Build history of the part. All positions in model axes, mm. A direction names the side the tool comes from. Round coordinates to 2 decimals unless told otherwise and drop trailing zeros. Loops run counter-clockwise (first coordinate to the right, second up) from the corner with the lowest first, then second, coordinate; pieces in that order, holes last.
from build123d import *

# Parameters (mm, degrees)
SALIENTE_EXTRUIR1_DEPTH = 304.8
CROQUIS4_R              = 15.875
SALIENTE_EXTRUIR2_DEPTH = 50.8
CROQUIS5_R              = 15.875
SALIENTE_EXTRUIR3_DEPTH = 25.4


with BuildPart() as part:
    # Croquis2 → Saliente-Extruir1 (new body)
    with BuildSketch(Plane.XY):
        Polygon((-63.5, 0), (-31.75, -54.99261314), (31.75, -54.99261314), (63.5, 0), (31.75, 54.99261314), (-31.75, 54.99261314), align=None)
    extrude(amount=-SALIENTE_EXTRUIR1_DEPTH)

    # Croquis4 → Saliente-Extruir2 (add)
    with BuildSketch(Plane.XY):
        Circle(CROQUIS4_R)
    extrude(amount=SALIENTE_EXTRUIR2_DEPTH)

    # Croquis5 → Saliente-Extruir3 (add)
    with BuildSketch(Plane(origin=(0, 0, -304.8), x_dir=(-1, 0, 0), z_dir=(0, 0, -1))):
        Circle(CROQUIS5_R)
    extrude(amount=SALIENTE_EXTRUIR3_DEPTH)


solid = part.part
(1) Slice it at B-B on z = -233. List the corners of the cut face in (x, y).
Responses:
outline: (-63.5, 0) - (-31.75, -54.99) - (31.75, -54.99) - (63.5, 0) - (31.75, 54.99) - (-31.75, 54.99) - close
(2) Slice it at A-A on x = 0. List the corners of the cut face in (y, z) (3 decimals), plus the area to 3 significant figures.
Responses:
outline: (-54.993, -304.8) - (-15.875, -304.8) - (-15.875, -330.2) - (15.875, -330.2) - (15.875, -304.8) - (54.993, -304.8) - (54.993, 0) - (15.875, 0) - (15.875, 50.8) - (-15.875, 50.8) - (-15.875, 0) - (-54.993, 0) - close
area: 35,900 mm2
(3) Slice it at C-C on y = 5.5. List the corners of the cut face in (x, z), plus the area to 3 significant figures.
Responses:
outline: (-60.32, -304.8) - (-14.89, -304.8) - (-14.89, -330.2) - (14.89, -330.2) - (14.89, -304.8) - (60.32, -304.8) - (60.32, 0) - (14.89, 0) - (14.89, 50.8) - (-14.89, 50.8) - (-14.89, 0) - (-60.32, 0) - close
area: 39,000 mm2
(4) Pin check, flat tips, straight feed: P1, Ø1.5, axis at y = 32, z = -75.5, coming from the +X side; P2, Ø1.5, axis at x = 36.5, z = -157.5, coming from the +Y side; P3, Ø5, axis at x = -35.5, y = -9, coming from the +Z side. Stop position of each tip, or through.
Responses:
P1: stops at x = 45.46
P2: stops at y = 48.06
P3: stops at z = 0
(5) Slice it at D-D on y = 43. List the corners of the cut face in (x, z), plus the area to 3 significant figures.
Responses:
outline: (-38.67, -304.8) - (38.67, -304.8) - (38.67, 0) - (-38.67, 0) - close
area: 23,600 mm2
(6) Probe line 1 (Z direction, x = -1, y = -35); line 2 (X direction, y = -8, z = -20.5); line 3 (X direction, y = 16, z = -93). List the from-to ranges inside material, lowest first.
Responses:
line 1: z = -304.8 to 0
line 2: x = -58.88 to 58.88
line 3: x = -54.26 to 54.26
(7) Which spindle directions (+Z, -Z, +X, -X, +Y, -Y) get a long thin tool onto all of the face, cutting with end or side? Do faces 1 (the face through (0, 54.993, -150)), 2 (the face through (3.441, -15.497, -317.322)), 3 (the face through (13, 13, 0)). Say none if no direction does.
Responses:
face 1: +Z, -Z, +X, -X, +Y
face 2: -Z
face 3: +Z
